Autodesk Inventor part; units mm, degrees
ref_plane "YZ Plane" through (0, 0, 0) normal (1, 0, 0) x (0, 1, 0)
ref_plane "XZ Plane" through (0, 0, 0) normal (0, 1, 0) x (-1, 0, 0)
ref_plane "XY Plane" through (0, 0, 0) normal (0, 0, 1) x (1, 0, 0)
sketch "Sketch1" plane through (0, 0, 0) normal (0, 1, 0) x (-1, 0, 0)
  line L0 (-4, 4.75) -> (4, 4.75)
  line L1 (4, 4.75) -> (4, -4.75)
  line L2 (4, -4.75) -> (-4, -4.75)
  line L3 (-4, -4.75) -> (-4, 4.75)
  line L4 (-4, 4.75) -> (4, -4.75) construction
  line L5 (4, 4.75) -> (-4, -4.75) construction
  point P0 (0, 0)
  dimension "d0" = 8
  dimension "d1" = 9.5
extrude "Extrusion1" add sketch "Sketch1" along normal blind 4
sketch "Sketch2" plane through (-4, 0, 4.75) normal (0, 0, 1) x (1, 0, 0)
  circle A0 centre (0, 0) radius 2
  circle A1 centre (8, 0) radius 2
  point P0 (4, 0)
  dimension "d4" = 4
  dimension "d5" = 4
extrude "Extrusion2" cut sketch "Sketch2" against normal blind 10
sketch "Sketch3" plane through (-4, 4, 4.75) normal (0, 0, 1) x (1, 0, 0)
  line L0 (0.3545, -0.2253) -> (7.5248, -0.2253)
  line L1 (7.5248, -0.2253) -> (7.5248, -1.7593)
  line L2 (7.5248, -1.7593) -> (0.3545, -1.7593)
  line L3 (0.3545, -1.7593) -> (0.3545, -0.2253)
  line L4 (2.5091, -3.2933) -> (5.3703, -3.2933)
  line L5 (5.3703, -3.2933) -> (5.3703, -0.2253)
  line L6 (5.3703, -0.2253) -> (2.5091, -0.2253)
  line L7 (2.5091, -0.2253) -> (2.5091, -3.2933)
  line L8 (2.5091, -3.2933) -> (5.3703, -0.2253) construction
  line L9 (5.3703, -3.2933) -> (2.5091, -0.2253) construction
  point P0 (4, -4)
  point P1 (3.9397, -1.7593)
extrude "Extrusion3" cut sketch "Sketch3" against normal blind 8
fillet "Fillet1" radius 2 2 edges at (-1.4909, 2.2407, 0.75) (1.3703, 2.2407, 0.75)
properties part number "USB-slot"
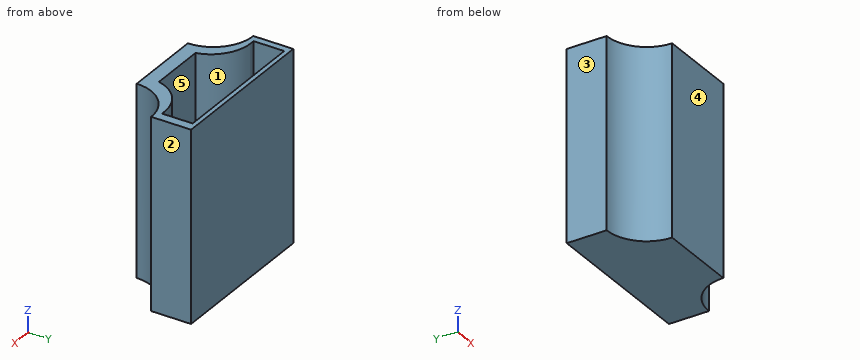
Geometry check sheet. Reference: the model listing, model coordinates, mm. Face numbers are marked on the shaded views. A direction names the side the tool comes from. Round coordinates to 2 decimals unless told otherwise and drop trailing zeros. Loops run counter-clockwise (first coordinate to the right, second up) from the corner with the lowest first, then second, coordinate; pieces in that order, holes last. Notation, with made-up numbers: M 70.25,-28 L 81.25,-28 A15 cw 81.25,-1 Z; hole C 6,77.25 d1. An arc over 180 degrees is marked long. Return JSON: item names as keys, results as strings. Group by question number.
(1) Section check D-D, the plane z = -3.5. Enter the section's corners in (x, y).
(2) Mould release check, pull along X, two halves, no side actions. Record for the marked faces 3, 4 and 5: pulls with the +X half, pulls with the -X half, needs draft (parallel to the pull), parting line crosses it, or undercut.
(3) Section check B-B, the plane x = 0.5. Enter the section's corners in (y, z), and give its area (3 significant figures).
(4) Scan lines: line 1 along X through (y, z) = (3.65, 2.25); line 2 along Y through (x, z) = (1, 4); line 3 along Z through (x, y) = (1.5, 1.5). Record each from-to range of solid material in increasing order. Write a range as [from, to].
(5) Section check A-A, the plane z = -1.25. Enter the section's corners in (x, y), and give its area (3 significant figures).
(6) Set-up check for the marked faces 1 and 2: record each of +Z, -Z, +X, -X, +Y, -Y from which the full face is reachable in a straight line by a thin tool's end or side.
(7) Section check C-C, the plane y = 2.35. Enter the section's corners in (x, z), and give its area (3 significant figures).
Data:
{
 "1": {"outline": "M -4,2 A2 cw -2,0 L 2,0 A2 cw 4,2 L 4,4 L -4,4 Z"},
 "2": {"face 3": "pulls with the -X half", "face 4": "needs draft", "face 5": "undercut"},
 "3": {"outline": "M 0,-4.75 L 4,-4.75 L 4,4.75 L 3.77,4.75 L 3.77,-3.25 L 0.71,-3.25 L 0.71,4.75 L 0,4.75 Z", "area": "13.5 mm²"},
 "4": {"line 1": "[-4, -3.65], [3.52, 4]", "line 2": "[0, 0.71], [3.77, 4]", "line 3": "[-4.75, -3.25]"},
 "5": {"outline": "M -4,2 A2 cw -2,0 L 2,0 A2 cw 4,2 L 4,4 L -4,4 Z; hole M -3.65,2.24 L -3.44,2.24 A2 cw -1.49,0.71 L 1.37,0.71 A2 cw 3.32,2.24 L 3.52,2.24 L 3.52,3.77 L -3.65,3.77 Z", "area": "8.80 mm²"},
 "6": {"face 1": "+Z", "face 2": "+Z, -Z, +X, +Y, -Y"},
 "7": {"outline": "M -4,-4.75 L 4,-4.75 L 4,4.75 L 3.52,4.75 L 3.52,-3.25 L -3.65,-3.25 L -3.65,4.75 L -4,4.75 Z", "area": "18.6 mm²"}
}
